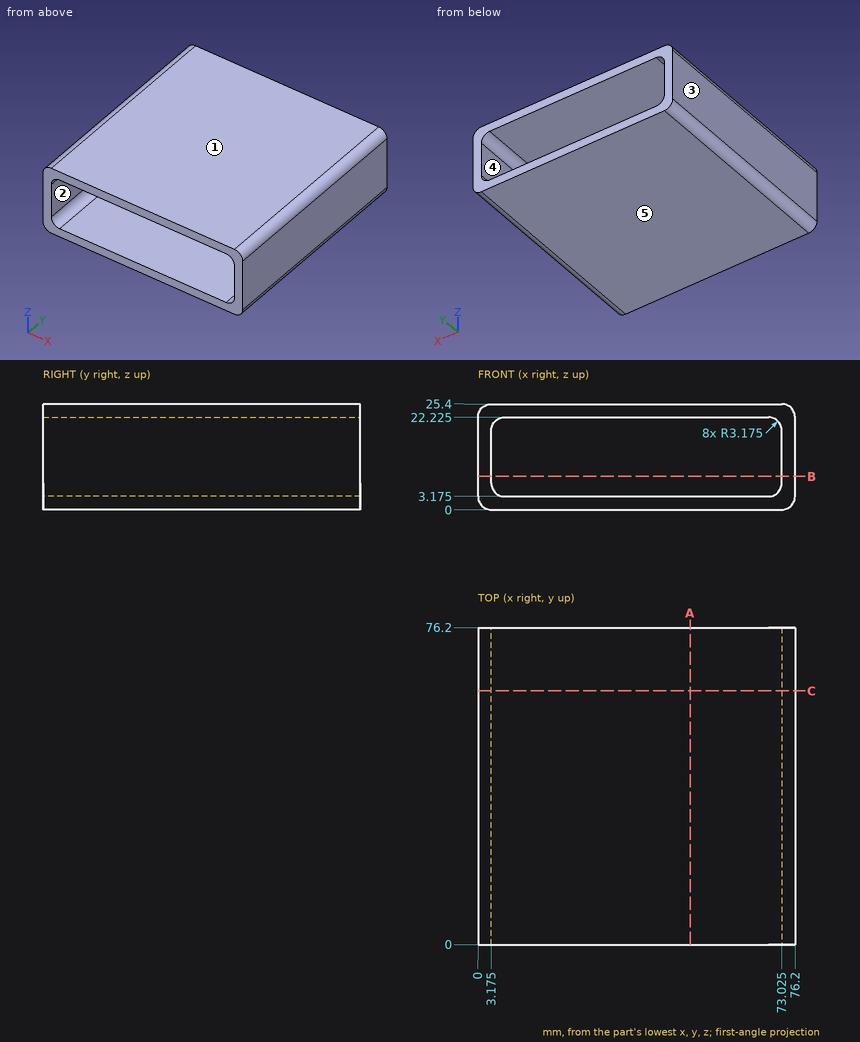
Design review of the part shown in the three views and the two pictorial views. Dimensions are in mm from the part's minimum x, y and z. A direction names the side the tool comes from. Give positions to 0.01 mm unless a question says otherwise; leave off trailing zeros. Write each loop counter-clockwise with the first axis right and the second up, starting at its lowest first coordinate (ties: lowest second). Pieces come first, ordered by that corner, then holes. Notation, with made-up numbers: M 63.25,31.25 L 71.25,31.25 A6 cw 71.25,37.25 Z; hole C 9.25,4 d1. An arc over 180 degrees is marked long. Answer as CSV lines item,"result".
1. Consider section A-A, the plane x = 51. Write out the cut boundary in (y, z) (3 decimals), then the cut area to 3 significant figures.
Findings:
outline,"M 0,0 L 76.2,0 L 76.2,3.175 L 0,3.175 Z; M 0,22.225 L 76.2,22.225 L 76.2,25.4 L 0,25.4 Z"
area,"484 mm2"
2. For the marked faces 1 and 2, list the 3-axis set-ups (+Z, -Z, +X, -X, +Y, -Y) from which the entire face can be reached by the end or side of a thin tool; tool diameter is ignored.
Findings:
face 1,"+Z, +X, -X, +Y, -Y"
face 2,"+Y, -Y"
3. Draft analysis for pull direction X (two halves, no side actions). For the marked faces 3, 4 and 5, state which applies: +X half, -X half, draft (parallel to the pull), parting line (faces both ways), or undercut.
Findings:
face 3,"-X half"
face 4,"undercut"
face 5,"draft"
4. Consider section B-B, the plane z = 8. Write out the cut boundary in (x, y) (3 decimals), then the cut area to 3 significant figures.
Findings:
outline,"M 0,0 L 3.175,0 L 3.175,76.2 L 0,76.2 Z; M 73.025,0 L 76.2,0 L 76.2,76.2 L 73.025,76.2 Z"
area,"484 mm2"
5. Wall thickness on line 1 (Z direction, x = 6, y = 19.5); line 2 (X direction, y = 12, z = 13.25) (3 decimals); line 3 (X direction, y = 36, z = 5.5): over which ranges is each line inside the solid? List them lowest first.
Findings:
line 1,"z = 0 to 3.19, 22.21 to 25.4"
line 2,"x = 0 to 3.175, 73.025 to 76.2"
line 3,"x = 0 to 3.29, 72.91 to 76.2"
6. Consider section C-C, the plane y = 61. Write out the cut boundary in (x, z) (3 decimals).
Findings:
outline,"M 0,3.175 A3.175 ccw 3.175,0 L 73.025,0 A3.175 ccw 76.2,3.175 L 76.2,22.225 A3.175 ccw 73.025,25.4 L 3.175,25.4 A3.175 ccw 0,22.225 Z; hole M 3.175,6.35 A3.175 ccw 6.35,3.175 L 69.85,3.175 A3.175 ccw 73.025,6.35 L 73.025,19.05 A3.175 ccw 69.85,22.225 L 6.35,22.225 A3.175 ccw 3.175,19.05 Z"
